Verification items for the finished model (mm, model axes). Face numbers are marked on the shaded views. A direction names the side the tool comes from. Give positions to 0.01 mm unless a question says otherwise; leave off trailing zeros. Loops run counter-clockwise (first coordinate to the right, second up) from the corner with the lowest first, then second, coordinate; pieces in that order, holes last. Notation, with made-up numbers: (1.25, 44.5) - (11.25, 44.5) arc R20 ccw to (11.25, 70.5) - close; hole circle Ø1 at (62.5, 41.5). An arc over 180 degrees is marked (long way). One line per question, with ' | ' between items. Start each with the question number.
1. Thickness scan on line 1 along X through (y, z) = (3.5, 0); line 2 along Z through (x, y) = (36, 1.5); line 3 along X through (y, z) = (1.5, -39). Record the ranges inside material, lowest first. Write a range as from..to.
2. Section check A-A, the plane x = -58. Enter the section's corners in (y, z).
3. Section check D-D, the plane x = 39. Enter the section's corners in (y, z), then the cut area to 3 significant figures.
4. Section check B-B, the plane y = 9.25. Enter the section's corners in (x, z) (1 decimal), then the cut area to 3 significant figures.
5. Depth check by flat-ended pin: pin 1 Ø5 at (y, z) = (5, -53.5) entering from -X; pin 2 Ø3 at (x, y) = (-47, 3) entering from +Z; pin 3 Ø1.5 at (y, z) = (8.5, 62) entering from -X. Enter the tip coordinate at first touch or a pass-through.
6. Section check C-C, the plane z = -56. Enter the section's corners in (x, y).
7. Tool access check on the marked faces 1 and 2. Record the directions out of +Z, -Z, +X, -X, +Y, -Y that give a thin tool (end or side, any length) a straight path to the whole face; none if there is none.
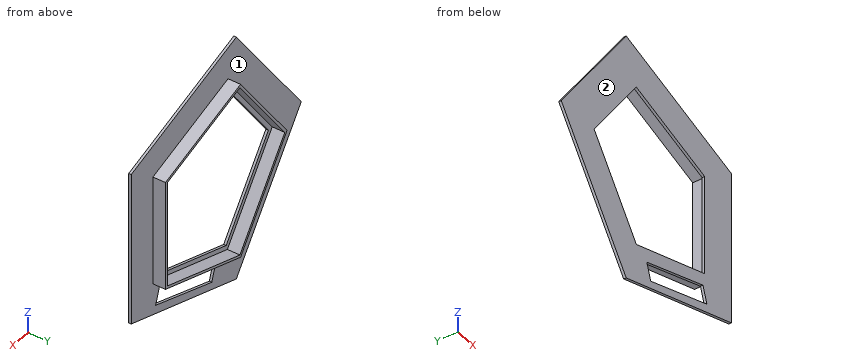
Autodesk Inventor part; units mm, degrees
ref_plane "YZ Plane" through (0, 0, 0) normal (1, 0, 0) x (0, 1, 0)
ref_plane "XZ Plane" through (0, 0, 0) normal (0, 1, 0) x (-1, 0, 0)
ref_plane "XY Plane" through (0, 0, 0) normal (0, 0, 1) x (1, 0, 0)
sketch "草图1" plane through (0, 0, 0) normal (0, 1, 0) x (-1, 0, 0)
  line L0 (68.3073, 0) -> (21.1081, -64.9641)
  line L1 (21.1081, -64.9641) -> (-55.2617, -40.15)
  line L2 (-55.2617, -40.15) -> (-55.2617, 40.15)
  line L3 (-55.2617, 40.15) -> (21.1081, 64.9641)
  line L4 (21.1081, 64.9641) -> (68.3073, 0)
  line L5 (105.0554, 0) -> (32.4639, -99.9136)
  line L6 (32.4639, -99.9136) -> (-84.9916, -61.75)
  line L7 (-84.9916, -61.75) -> (-84.9916, 61.75)
  line L8 (-84.9916, 61.75) -> (32.4639, 99.9136)
  line L9 (32.4639, 99.9136) -> (105.0554, 0)
  point P0 (0, 0)
  point P1 (0, 0)
  point P2 (0, 0)
  dimension "d0" = 80.3
  dimension "d1" = 123.5
extrude "拉伸1" add sketch "草图1" along normal blind 2
sketch "草图2" plane through (0, 2, 0) normal (0, 1, 0) x (1, 0, 0)
  line L0 (-21.1081, 64.9641) -> (55.2617, 40.15)
  line L1 (55.2617, 40.15) -> (55.2617, -40.15)
  line L2 (55.2617, -40.15) -> (-21.1081, -64.9641)
  line L3 (-21.1081, -64.9641) -> (-68.3073, 0)
  line L4 (-68.3073, 0) -> (-21.1081, 64.9641)
  line L5 (-32.4639, 99.9136) -> (-105.0554, 0)
  line L6 (-105.0554, 0) -> (-32.4639, -99.9136)
  line L7 (-32.4639, -99.9136) -> (84.9916, -61.75)
  line L8 (84.9916, -61.75) -> (84.9916, 61.75)
  line L9 (84.9916, 61.75) -> (-32.4639, 99.9136)
  line L10 (58.7617, 42.6929) -> (-22.445, 69.0786)
  line L11 (-22.445, 69.0786) -> (-72.6335, 0)
  line L12 (-72.6335, 0) -> (-22.445, -69.0786)
  line L13 (-22.445, -69.0786) -> (58.7617, -42.6929)
  line L14 (58.7617, -42.6929) -> (58.7617, 42.6929)
  line L15 (-23.2089, 71.4297) -> (60.7617, 44.146)
  line L16 (60.7617, 44.146) -> (60.7617, -44.146)
  line L17 (60.7617, -44.146) -> (-23.2089, -71.4297)
  line L18 (-23.2089, -71.4297) -> (-75.1056, 0)
  line L19 (-75.1056, 0) -> (-23.2089, 71.4297)
  point P0 (0, 0)
  dimension "d4" = 3.5
  dimension "d5" = 2
extrude "拉伸2" add sketch "草图2" along normal blind 10 contours L15 L16 L17 L18 L19
sketch "草图3" plane through (0, 0, 0) normal (0, -1, 0) x (1, 0, 0)
  line L0 (-9.4145, -72.1274) -> (53.3776, -50.8644)
  line L1 (53.3776, -50.8644) -> (57.7542, -63.7889)
  line L2 (57.7542, -63.7889) -> (-5.038, -85.0518)
  line L3 (-5.038, -85.0518) -> (-9.4145, -72.1274)
  point P0 (0, 0)
extrude "拉伸3" cut sketch "草图3" against normal blind 10
properties part number "上部端盖" material "ABS 塑料"
Results list:
1) line 1: -75.11..-72.63, 58.76..60.76 | line 2: -77.67..-71.16, -56.75..-46.41, 46.41..77.67 | line 3: -76.72..-39.97, 55.26..84.99
2) outline: (0, -64.77) - (2, -64.77) - (2, -23.54) - (12, -23.54) - (12, -20.14) - (2, -20.14) - (2, -14.19) - (0, -14.19) - close; (0, 14.19) - (2, 14.19) - (2, 20.14) - (12, 20.14) - (12, 23.54) - (2, 23.54) - (2, 64.77) - (0, 64.77) - close
3) outline: (0, -76.69) - (2, -76.69) - (2, -70.14) - (0, -70.14) - close; (0, -55.73) - (2, -55.73) - (2, -51.22) - (12, -51.22) - (12, -49.11) - (2, -49.11) - (2, -45.43) - (0, -45.43) - close; (0, 45.43) - (2, 45.43) - (2, 49.11) - (12, 49.11) - (12, 51.22) - (2, 51.22) - (2, 76.69) - (0, 76.69) - close | area: 138 mm²
4) outline: (-75.1, 0) - (-23.2, -71.4) - (60.8, -44.1) - (60.8, 44.1) - (-23.2, 71.4) - close; hole (-72.6, 0) - (-22.4, -69.1) - (58.8, -42.7) - (58.8, 42.7) - (-22.4, 69.1) - close | area: 868 mm²
5) pin 1: x = -38.05 | pin 2: z = 81.45 | pin 3: x = -30.6
6) outline: (-64.37, 0) - (-27.62, 0) - (-27.62, 2) - (-31.95, 2) - (-31.95, 12) - (-34.42, 12) - (-34.42, 2) - (-64.37, 2) - close; (6.48, 0) - (38.21, 0) - (38.21, 2) - (24.28, 2) - (24.28, 12) - (17.81, 12) - (17.81, 2) - (6.48, 2) - close; (55.12, 0) - (84.99, 0) - (84.99, 2) - (55.12, 2) - close
7) face 1: +Y | face 2: +Z, -Z, +X, -X, -Y
